Input: part model. Units: mm. Frame: model coordinates. Round coordinates to 2 decimals unless told otherwise and drop trailing zeros. Order: outer loops, then holes, each group sorted by start corner. A loop starts at its lowest first (then second) coordinate and runs counter-clockwise, first axis right, second up.
Item 1: Cut plane C-C on y = -46. Output: boundary loops of the cut face in (x, z), then the cut area to 3 significant figures.
Item 2: First-contact query: pin 1 (2 mm diameter, centred on y = -81.52, z = 97.9, fed in from +X); pin 2 (1.5 mm diameter, centred on x = 3.5, z = 149.5, fed in from -Y); pin 3 (1.2 mm diameter, centred on x = 1.5, y = -189, fed in from -Z). Flat tips, straight axial feed; report the tip coordinate or a pass-through.
Item 3: Cut plane B-B on z = 75.5. Output: boundary loops of the cut face in (x, y), then the cut area to 3 significant figures.
Item 4: Cut plane D-D on z = 58. Output: boundary loops of the cut face in (x, y), then the cut area to 3 significant figures.
Item 5: Line query: L1, parallel to Z at x = 1.5, y = -82; L2, parallel to Z at x = 0.55, y = -128; L3, parallel to Z at x = 0.35, y = -98.5. Output: solid intervals per line, ascending.
Item 6: Cut plane A-A on x = 0.95. Give the number of separate pieces and of enclosed holes in the cut face, then the cut area to 3 significant figures.
```python
from build123d import *

# Parameters (mm, degrees)
AUFSATZ_LINEAR_AUSTRAGEN1_DEPTH      = 4
SKIZZE1_9_R                          = 10
SCHNITT_LINEAR_AUSTRAGEN1_DEPTH      = 6
SCHNITT_LINEAR_AUSTRAGEN2_DEPTH      = 251.325290812
SCHNITT_LINEAR_AUSTRAGEN2_DEPTH_BACK = 10
M3_GEWINDEBOHRUNG1_D                 = 2.5
M3_GEWINDEBOHRUNG1_DEPTH             = 8.5
M3_GEWINDEBOHRUNG1_TIP               = 0.751075774
KREISMUSTER1_COUNT                   = 4
DURCHGANGSLOCH_F_R_M61_D             = 6.6
DURCHGANGSLOCH_F_R_M61_DEPTH         = 17
DURCHGANGSLOCH_F_R_M61_TIP           = 1.982840043
SKIZZE32_W                           = 4
SKIZZE32_H                           = 30
AUFSATZ_LINEAR_AUSTRAGEN2_DEPTH      = 4


with BuildPart() as part:
    # Skizze1 → Aufsatz-Linear austragen1 (new body)
    with BuildSketch(Plane(origin=(0, 0, 0), x_dir=(0, 0, -1), z_dir=(1, 0, 0))):
        with BuildLine():
            Line((-120.903454086, -13.395859459), (-120.903454086, -24.075118314))
            ThreePointArc((-120.903454086, -24.075118314), (-140.453351678, -44.726591756), (-150.175306123, -71.450465968))
            Line((-150.175306123, -71.450465968), (-166.903454086, -186.520744783))
            Line((-166.903454086, -186.520744783), (-10.903454086, -186.520744783))
            Line((-10.903454086, -186.520744783), (-1.903454086, -186.520744783))
            Line((-1.903454086, -186.520744783), (-1.903454086, -81.52074478))
            ThreePointArc((-1.903454086, -81.52074478), (-41.654250272, -12.960552248), (-120.903454086, -13.395859459))
        make_face()
    extrude(amount=AUFSATZ_LINEAR_AUSTRAGEN1_DEPTH)

    # Skizze1<9> → Schnitt-Linear austragen1 (cut)
    with BuildSketch(Plane(origin=(0, 0, 0), x_dir=(0, 0, -1), z_dir=(1, 0, 0))):
        with Locations((-80.903454086, -81.52074478)):
            Circle(SKIZZE1_9_R)
    extrude(amount=SCHNITT_LINEAR_AUSTRAGEN1_DEPTH, mode=Mode.SUBTRACT)

    # Skizze3 → Durchgangsloch für M31 (revolve, cut)
    with BuildSketch(Plane(origin=(0, -81.52074478, 63.903454086), x_dir=(0, 0, 1), z_dir=(0, 1, 0))):
        Polygon((0, 0), (0, 21.021463052), (1.7, 20), (1.7, 0), align=None)
    durchgangsloch_f_r_m31 = revolve(axis=Axis((-6.35, -81.52074478, 63.903454086), (1, 0, 0)), mode=Mode.SUBTRACT)

    # Skizze1<18> → Schnitt-Linear austragen2 (cut, two sides: drawn at the far end of the back side and taken through both)
    with BuildSketch(Plane(origin=(0, 0, 0), x_dir=(0, 0, -1), z_dir=(1, 0, 0)).offset(-SCHNITT_LINEAR_AUSTRAGEN2_DEPTH_BACK)):
        with BuildLine():
            ThreePointArc((-1.903454086, -81.52074478), (-41.654250272, -12.960552248), (-120.903454086, -13.395859459))
            Line((-120.903454086, -13.395859459), (-120.903454086, -24.075118314))
            ThreePointArc((-120.903454086, -24.075118314), (-48.499750594, -19.47237655), (-10.903454086, -81.52074478))
            Line((-10.903454086, -81.52074478), (-10.903454086, -186.520744783))
            Line((-10.903454086, -186.520744783), (-1.903454086, -186.520744783))
            Line((-1.903454086, -186.520744783), (-1.903454086, -81.52074478))
        make_face()
    extrude(amount=SCHNITT_LINEAR_AUSTRAGEN2_DEPTH + SCHNITT_LINEAR_AUSTRAGEN2_DEPTH_BACK, mode=Mode.SUBTRACT)

    # M3 Gewindebohrung1
    with Locations(Plane.YZ.offset(4)):
        with Locations((-176.520744783, 14.903454086), (-126.520744783, 14.903454086), (-34.851697221, 34.234406527), (-19.501031808, 103.476783545), (-81.52074478, 14.903454086), (-72.025910472, 146.216914578), (-126.520744783, 154.139009327)):
            Hole(M3_GEWINDEBOHRUNG1_D / 2, depth=M3_GEWINDEBOHRUNG1_DEPTH)
            with Locations((0, 0, -(M3_GEWINDEBOHRUNG1_DEPTH + M3_GEWINDEBOHRUNG1_TIP / 2))):  # 118° drill point
                Cone(0, M3_GEWINDEBOHRUNG1_D / 2, M3_GEWINDEBOHRUNG1_TIP, mode=Mode.SUBTRACT)

    # Kreismuster1: Durchgangsloch für M31 ×4 about axis
    kreismuster1_axis = Axis((0, -81.52074478, 80.903454086), (1, 0, 0))
    for i in range(1, KREISMUSTER1_COUNT):
        add(durchgangsloch_f_r_m31.rotate(kreismuster1_axis, i * 360 / KREISMUSTER1_COUNT), mode=Mode.SUBTRACT)

    # Durchgangsloch für M61
    with Locations(Plane.ZY):
        with Locations((40.903454086, -126.520744783), (125.903454086, -126.520744783)):
            Hole(DURCHGANGSLOCH_F_R_M61_D / 2, depth=DURCHGANGSLOCH_F_R_M61_DEPTH)
            with Locations((0, 0, -(DURCHGANGSLOCH_F_R_M61_DEPTH + DURCHGANGSLOCH_F_R_M61_TIP / 2))):  # 118° drill point
                Cone(0, DURCHGANGSLOCH_F_R_M61_D / 2, DURCHGANGSLOCH_F_R_M61_TIP, mode=Mode.SUBTRACT)

    # Skizze32 → Aufsatz-Linear austragen2 (add)
    with BuildSketch(Plane.XZ.offset(186.520744783)):
        with Locations((2, 119.903454086)):
            Rectangle(SKIZZE32_W, SKIZZE32_H)
        with Locations((2, 57.903454086)):
            Rectangle(SKIZZE32_W, SKIZZE32_H)
    extrude(amount=AUFSATZ_LINEAR_AUSTRAGEN2_DEPTH)


solid = part.part
```
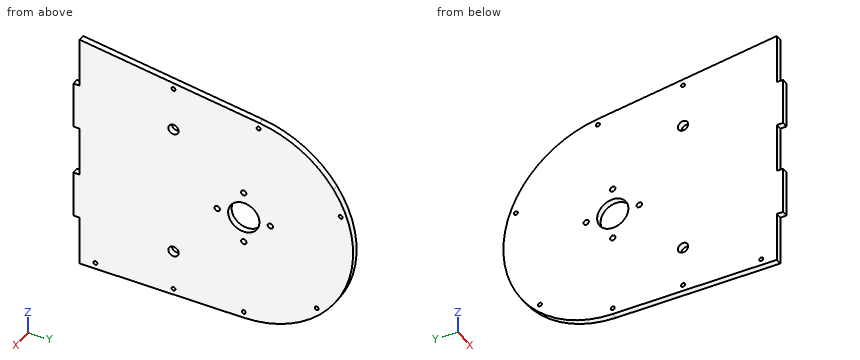
From the geometry:
1. outline: (0, 20.59) - (4, 20.59) - (4, 141.22) - (0, 141.22) - close
1. area: 483 mm2
2. pin 1: passes through
2. pin 2: stops at y = -186.52
2. pin 3: stops at z = 42.9
3. outline: (0, -186.52) - (4, -186.52) - (4, -89.94) - (0, -89.94) - close; (0, -73.11) - (4, -73.11) - (4, -11.73) - (0, -11.73) - close
3. area: 632 mm2
4. outline: (0, -190.52) - (4, -190.52) - (4, -15.37) - (0, -15.37) - close
4. area: 701 mm2
5. L1: z = 10.9 to 13.75, 16.06 to 62.27, 65.53 to 70.91, 90.89 to 96.27, 99.53 to 151.71
5. L2: z = 10.9 to 37.95, 43.85 to 122.95, 128.85 to 158.4
5. L3: z = 10.9 to 79.2, 82.6 to 154.11
6. separate pieces: 1
6. enclosed holes: 14
6. area: 23,100 mm2
